```python
from build123d import *

# Parameters (mm, degrees)
SKETCH1_R           = 4
SKETCH1_R_2         = 3.5
BOSS_EXTRUDE1_DEPTH = 5
BOSS_EXTRUDE2_START = -5
SKETCH1_3_R         = 4
BOSS_EXTRUDE2_DEPTH = 10.6
BOSS_EXTRUDE3_START = -15.6
SKETCH1_4_R         = 4
SKETCH1_4_R_2       = 3.5
BOSS_EXTRUDE3_DEPTH = 5


with BuildPart() as part:
    # Sketch1 → Boss-Extrude1 (new body)
    # profile 1 of 2: a face of its own
    with BuildSketch(Plane.XY):
        with BuildLine():
            Line((-25, -36.3), (25, -36.3))
            ThreePointArc((25, -36.3), (32.292866569, -31.588479467), (30.995610492, -23.003524301))
            ThreePointArc((30.995610492, -23.003524301), (28.288479467, -21.007133431), (25, -20.3))
            Line((25, -20.3), (-25, -20.3))
            ThreePointArc((-25, -20.3), (-28.288479467, -21.007133431), (-30.995610492, -23.003524301))
            ThreePointArc((-30.995610492, -23.003524301), (-32.292866569, -31.588479467), (-25, -36.3))
        make_face()
        with Locations((-25, -28.3)):
            Circle(SKETCH1_R, mode=Mode.SUBTRACT)
        with Locations((25, -28.3)):
            Circle(SKETCH1_R, mode=Mode.SUBTRACT)
    # profile 2 of 2: a face of its own
    with BuildSketch(Plane.XY):
        with BuildLine():
            ThreePointArc((25, -20.3), (28.288479467, -21.007133431), (30.995610492, -23.003524301))
            Line((30.995610492, -23.003524301), (5.995610492, 5.296475699))
            ThreePointArc((5.995610492, 5.296475699), (0, 8), (-5.995610492, 5.296475699))
            Line((-5.995610492, 5.296475699), (-30.995610492, -23.003524301))
            ThreePointArc((-30.995610492, -23.003524301), (-28.288479467, -21.007133431), (-25, -20.3))
            Line((-25, -20.3), (25, -20.3))
        make_face()
        Circle(SKETCH1_R_2, mode=Mode.SUBTRACT)
    extrude(amount=-BOSS_EXTRUDE1_DEPTH)

    # Sketch1<3> → Boss-Extrude2 (add)
    with BuildSketch(Plane.XY.offset(BOSS_EXTRUDE2_START)):
        with BuildLine():
            Line((-25, -36.3), (25, -36.3))
            ThreePointArc((25, -36.3), (32.292866569, -31.588479467), (30.995610492, -23.003524301))
            ThreePointArc((30.995610492, -23.003524301), (28.288479467, -21.007133431), (25, -20.3))
            Line((25, -20.3), (-25, -20.3))
            ThreePointArc((-25, -20.3), (-28.288479467, -21.007133431), (-30.995610492, -23.003524301))
            ThreePointArc((-30.995610492, -23.003524301), (-32.292866569, -31.588479467), (-25, -36.3))
        make_face()
        with Locations((-25, -28.3)):
            Circle(SKETCH1_3_R, mode=Mode.SUBTRACT)
        with Locations((25, -28.3)):
            Circle(SKETCH1_3_R, mode=Mode.SUBTRACT)
    extrude(amount=-BOSS_EXTRUDE2_DEPTH)

    # Sketch1<4> → Boss-Extrude3 (add)
    # profile 1 of 2: a face of its own
    with BuildSketch(Plane.XY.offset(BOSS_EXTRUDE3_START)):
        with BuildLine():
            Line((-25, -36.3), (25, -36.3))
            ThreePointArc((25, -36.3), (32.292866569, -31.588479467), (30.995610492, -23.003524301))
            ThreePointArc((30.995610492, -23.003524301), (28.288479467, -21.007133431), (25, -20.3))
            Line((25, -20.3), (-25, -20.3))
            ThreePointArc((-25, -20.3), (-28.288479467, -21.007133431), (-30.995610492, -23.003524301))
            ThreePointArc((-30.995610492, -23.003524301), (-32.292866569, -31.588479467), (-25, -36.3))
        make_face()
        with Locations((-25, -28.3)):
            Circle(SKETCH1_4_R, mode=Mode.SUBTRACT)
        with Locations((25, -28.3)):
            Circle(SKETCH1_4_R, mode=Mode.SUBTRACT)
    # profile 2 of 2: a face of its own
    with BuildSketch(Plane.XY.offset(BOSS_EXTRUDE3_START)):
        with BuildLine():
            ThreePointArc((25, -20.3), (28.288479467, -21.007133431), (30.995610492, -23.003524301))
            Line((30.995610492, -23.003524301), (5.995610492, 5.296475699))
            ThreePointArc((5.995610492, 5.296475699), (0, 8), (-5.995610492, 5.296475699))
            Line((-5.995610492, 5.296475699), (-30.995610492, -23.003524301))
            ThreePointArc((-30.995610492, -23.003524301), (-28.288479467, -21.007133431), (-25, -20.3))
            Line((-25, -20.3), (25, -20.3))
        make_face()
        Circle(SKETCH1_4_R_2, mode=Mode.SUBTRACT)
    extrude(amount=-BOSS_EXTRUDE3_DEPTH)


solid = part.part
```
For this review, take the finished solid that the model builds, in its own axes (mm). A direction names the side the tool comes from. Give positions to 0.01 mm unless a question says otherwise; leave off trailing zeros. Write each loop counter-clockwise with the first axis right and the second up, starting at its lowest first coordinate (ties: lowest second). Pieces come first, ordered by that corner, then holes. Notation, with made-up numbers: M 62,24.5 L 93,24.5 A24 ccw 93,47.5 Z; hole C -23,-23 d7. An arc over 180 degrees is marked long. Answer as CSV lines item,"result".
1. For faces 5 (the cylindrical face through (0, 8, -18)), 6 (the cylindrical face through (-32.998, -28.124, -10.156)), 7 (the cylindrical face through (32.998, -28.476, -10.156)), list the 3-axis set-ups (+Z, -Z, +X, -X, +Y, -Y) from which the entire face can be reached by the end or side of a thin tool; tool diameter is ignored.
Findings:
face 5,"+Z, -Z, +Y"
face 6,"-X"
face 7,"+X"
2. Consider section C-C, the plane z = -1.25. Write out the cut boundary in (x, y).
Findings:
outline,"M -31,-23 A8 ccw -25,-36.3 L 25,-36.3 A8 ccw 31,-23 L 6,5.3 A8 ccw -6,5.3 Z; hole C -25,-28.3 d8; hole C 0,0 d7; hole C 25,-28.3 d8"
3. For pin 1 (5.5 mm diameter, centred on x = 5, z = -12.5, fed in from +Y); pin 2 (6.5 mm diameter, centred on x = -25, y = -28.3, fed in from -Z); pin 3 (4 mm diameter, centred on x = -20, z = -4.5, fed in from +Y); pin 4 (5 mm diameter, centred on y = -2.5, z = -3, fed in from +X), all flat-tipped, find the tip position at first contact; note any pin that passes through.
Findings:
pin 1,"stops at y = -20.3"
pin 2,"passes through"
pin 3,"stops at y = -8.29"
pin 4,"stops at x = 15.09"
4. Consider section D-D, the plane y = -10. Write out the cut boundary in (x, z), then the cut area to 3 significant figures.
Findings:
outline,"M -19.51,-20.6 L 19.51,-20.6 L 19.51,-15.6 L -19.51,-15.6 Z; M -19.51,-5 L 19.51,-5 L 19.51,0 L -19.51,0 Z"
area,"390 mm2"
5. Draft analysis for pull direction Z (two halves, no side actions). For faces 1 (the flat face through (-18.321, -8.655, -2.465)), 2 (the flat face through (0, -20.3, -10)), 3 (the flat face through (0, -19, -20.6)), 4 (the flat face through (0, -11, -5)), state which applies: +Z half, -Z half, draft (parallel to the pull), parting line (faces both ways), or undercut.
Findings:
face 1,"draft"
face 2,"undercut"
face 3,"-Z half"
face 4,"undercut"
6. Wall thickness on line 1 (Z direction, x = -14, y = -8.5); line 2 (Y direction, x = 25, z = -15.5); line 3 (X direction, y = -26, z = -2.5): over which ranges is each line inside the solid? List them lowest first.
Findings:
line 1,"z = -20.6 to -15.6, -5 to 0"
line 2,"y = -36.3 to -32.3, -24.3 to -20.3"
line 3,"x = -32.66 to -28.27, -21.73 to 21.73, 28.27 to 32.66"
7. Consider section B-B, the plane y = -28.3. Write out the cut boundary in (x, z).
Findings:
outline,"M -33,-20.6 L -29,-20.6 L -29,0 L -33,0 Z; M -21,-20.6 L 21,-20.6 L 21,0 L -21,0 Z; M 29,-20.6 L 33,-20.6 L 33,0 L 29,0 Z"
8. Consider section A-A, the plane x = 0. Write out the cut boundary in (y, z).
Findings:
outline,"M -36.3,-20.6 L -3.5,-20.6 L -3.5,-15.6 L -20.3,-15.6 L -20.3,-5 L -3.5,-5 L -3.5,0 L -36.3,0 Z; M 3.5,-20.6 L 8,-20.6 L 8,-15.6 L 3.5,-15.6 Z; M 3.5,-5 L 8,-5 L 8,0 L 3.5,0 Z"
